from build123d import *

# Parameters (mm, degrees)
SKETCH2_R           = 105
SKETCH2_R_2         = 21.75
SKETCH2_R_3         = 5
SKETCH2_R_4         = 2
BOSS_EXTRUDE2_DEPTH = 3.175
SKETCH8_W           = 3.2
SKETCH8_H           = 6.353
CUT_EXTRUDE1_DEPTH  = 4.175
SKETCH9_R           = 1.5875
CUT_EXTRUDE2_DEPTH  = 4.175


with BuildPart() as part:
    # Sketch2 → Boss-Extrude2 (new body)
    with BuildSketch(Plane(origin=(0, 0, 0), x_dir=(1, 0, 0), z_dir=(0, 1, 0))):
        Circle(SKETCH2_R)
        with Locations((0, 80)):
            Circle(SKETCH2_R_2, mode=Mode.SUBTRACT)
        Circle(SKETCH2_R_3, mode=Mode.SUBTRACT)
        with Locations((17.5, 4.5)):
            Circle(SKETCH2_R_4, mode=Mode.SUBTRACT)
        with Locations((-17.5, 4.5)):
            Circle(SKETCH2_R_4, mode=Mode.SUBTRACT)
    extrude(amount=BOSS_EXTRUDE2_DEPTH)

    # Sketch8 → Cut-Extrude1 (cut, through all)
    with BuildSketch(Plane(origin=(0, 3.175, 0), x_dir=(1, 0, 0), z_dir=(0, 1, 0))):
        Polygon((-74.777, 57.507097448), (-71.577, 57.507096503), (-71.577, 44.804096503), (-74.777, 44.804095482), align=None)
        with Locations((73.177, -11.5824036)):
            Rectangle(SKETCH8_W, SKETCH8_H)
        Polygon((-74.777, 35.536096628), (-71.577, 35.536096628), (-71.577, 22.833096628), (-74.777, 22.833096317), align=None)
        Polygon((-74.777, 13.565096577), (-71.577, 13.565096577), (-71.577, 0.862096577), (-74.777, 0.862095696), align=None)
        with Locations((-73.177, -11.5824036)):
            Rectangle(SKETCH8_W, SKETCH8_H)
        Polygon((71.577, 13.565096577), (71.577, 0.862096577), (74.777, 0.862095696), (74.777, 13.565096577), align=None)
        Polygon((71.577, 35.536096628), (71.577, 22.833096628), (74.777, 22.833096317), (74.777, 35.536096628), align=None)
        Polygon((71.577, 57.507096503), (71.577, 44.804096503), (74.777, 44.804095482), (74.777, 57.507097448), align=None)
    extrude(amount=-CUT_EXTRUDE1_DEPTH, mode=Mode.SUBTRACT)

    # Sketch9 → Cut-Extrude2 (cut, through all)
    with BuildSketch(Plane.XZ):
        with Locations((51.250084, 2.0166)):
            Circle(SKETCH9_R)
        with Locations((-51.315116, -36.0326)):
            Circle(SKETCH9_R)
        with Locations((-51.250084, 2.0166)):
            Circle(SKETCH9_R)
        with Locations((51.315116, -36.0326)):
            Circle(SKETCH9_R)
    extrude(amount=-CUT_EXTRUDE2_DEPTH, mode=Mode.SUBTRACT)


solid = part.part
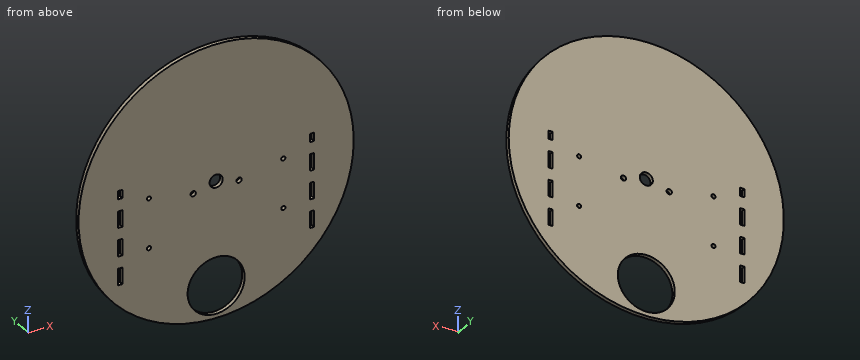
Part model, mm, in its own coordinate system. Give positions to 0.01 mm unless a question says otherwise; leave off trailing zeros. Loops run counter-clockwise (first coordinate to the right, second up) from the corner with the lowest first, then second, coordinate; pieces in that order, holes last. Notation, with made-up numbers: M 42,36 L 80,36 A17 cw 80,54 Z; hole C -30.5,35 d8. An arc over 180 degrees is marked long. Put each result on its own line as item: value. Start each with the question number.
1) Saw through at D-D (x = 65.5). List the corners of the cut face in (y, z) (3 decimals).
2) Saw through at B-B (z = -80). List the corners of the cut face in (x, y) (3 decimals), then the cut area to 3 significant figures.
3) Saw through at C-C (y = 1.95). State how many separate pieces and enclosed holes the cut face has, then the cut area to 3 significant figures.
4) Saw through at A-A (z = -10.5). List the corners of the cut face in (x, y) (3 decimals), then the cut area to 3 significant figures.
5) Probe probe 1 along X at (y, z) = (0.6, -4.5); probe 2 along Z at (x, y) = (-3, 0.25); probe 3 along Z at (x, y) = (19, 1.8). List the from-to ranges inside material, lowest first.
6) Flat gauge pins, fed straight in: pin 1 (1 mm diameter, centred on x = -72.5, y = 1, fed in from -Z); pin 2 (1 mm diameter, centred on y = 1.5, z = 12, fed in from +X); pin 3 (1.6 mm diameter, centred on y = 1, z = -7.5, fed in from +X). Where does each tip first touch, or does it go through?
Numbers:
1. outline: M 0,-82.066 L 3.175,-82.066 L 3.175,82.066 L 0,82.066 Z
2. outline: M -68.007,0 L -21.75,0 L -21.75,3.175 L -68.007,3.175 Z; M 21.75,0 L 68.007,0 L 68.007,3.175 L 21.75,3.175 Z
2. area: 294 mm^2
3. separate pieces: 1
3. enclosed holes: 16
3. area: 32,700 mm^2
4. outline: M -104.474,0 L -74.777,0 L -74.777,3.175 L -104.474,3.175 Z; M -71.577,0 L 71.577,0 L 71.577,3.175 L -71.577,3.175 Z; M 74.777,0 L 104.474,0 L 104.474,3.175 L 74.777,3.175 Z
4. area: 643 mm^2
5. probe 1: -104.9 to -74.78, -71.58 to -19.5, -15.5 to -2.18, 2.18 to 15.5, 19.5 to 71.58, 74.78 to 104.9
5. probe 2: -104.96 to -101.54, -58.46 to -4, 4 to 104.96
5. probe 3: -103.27 to -90.59, -69.41 to -5.82, -3.18 to 103.27
6. pin 1: z = -76.43
6. pin 2: x = 104.37
6. pin 3: x = 104.79
